from build123d import *

# Parameters (mm, degrees)
ESBO_O1_W                = 18
ESBO_O1_H                = 35
RESSALTO_EXTRUS_O1_DEPTH = 1.5
CORTE_EXTRUS_O1_REACH    = 21.906
ESBO_O2_W                = 13
ESBO_O2_H                = 23
CORTE_EXTRUS_O2_REACH    = 21.906
ESBO_O3_R                = 0.85
FILETE1_R                = 2
ESBO_O4_W                = 3
ESBO_O4_H                = 10
RESSALTO_EXTRUS_O2_DEPTH = 5.73
RESSALTO_EXTRUS_O2_DRAFT = -8
ESBO_O5_W                = 18.610597966
ESBO_O5_H                = 11.610597966
RESSALTO_EXTRUS_O3_DEPTH = 2
CORTE_EXTRUS_O4_REACH    = 46.648
ESBO_O7_R                = 1.75


with BuildPart() as part:
    # Esboço1 → Ressalto-extrusão1 (new, symmetric)
    with BuildSketch(Plane(origin=(0, 0, 0), x_dir=(0, 0, -1), z_dir=(1, 0, 0))):
        Rectangle(ESBO_O1_W, ESBO_O1_H)
    extrude(amount=RESSALTO_EXTRUS_O1_DEPTH, both=True)

    # Esboço2 → Corte-extrusão1 (cut, up to next)
    with BuildSketch(Plane(origin=(1.5, 0, 0), x_dir=(0, 0, -1), z_dir=(1, 0, 0)), mode=Mode.PRIVATE) as corte_extrus_o1_sk1:
        Rectangle(ESBO_O2_W, ESBO_O2_H)
    corte_extrus_o1_tool1 = extrude(corte_extrus_o1_sk1.sketch, amount=-CORTE_EXTRUS_O1_REACH, mode=Mode.PRIVATE) & part.part
    add(corte_extrus_o1_tool1.solids().sort_by_distance((1.5, 0, 0))[0], mode=Mode.SUBTRACT)

    # Esboço3 → Corte-extrusão2 (cut, up to next)
    with BuildSketch(Plane.ZY.offset(1.5), mode=Mode.PRIVATE) as corte_extrus_o2_sk1:
        with Locations((0, 14)):
            Circle(ESBO_O3_R)
    corte_extrus_o2_tool1 = extrude(corte_extrus_o2_sk1.sketch, amount=-CORTE_EXTRUS_O2_REACH, mode=Mode.PRIVATE) & part.part
    # Esboço3 → Corte-extrusão2 (cut, up to next)
    with BuildSketch(Plane.ZY.offset(1.5), mode=Mode.PRIVATE) as corte_extrus_o2_sk2:
        with Locations((0, -14)):
            Circle(ESBO_O3_R)
    corte_extrus_o2_tool2 = extrude(corte_extrus_o2_sk2.sketch, amount=-CORTE_EXTRUS_O2_REACH, mode=Mode.PRIVATE) & part.part
    add(corte_extrus_o2_tool1.solids().sort_by_distance((-1.5, 14, 0))[0], mode=Mode.SUBTRACT)
    add(corte_extrus_o2_tool2.solids().sort_by_distance((-1.5, -14, 0))[0], mode=Mode.SUBTRACT)

    # Filete1
    filete1_edges = [part.edges().sort_by_distance(p)[0] for p in [
        (0, -17.5, -9),
        (0, -17.5, 9),
        (0, 17.5, 9),
        (0, 17.5, -9),
    ]]
    fillet(filete1_edges, radius=FILETE1_R)


with BuildPart() as ressalto_extrus_o2_tool:
    # Esboço4 → Ressalto-extrusão2 (with draft: the straight prism first)
    with BuildSketch(Plane.XZ.offset(17.5)):
        Rectangle(ESBO_O4_W, ESBO_O4_H)
    extrude(amount=RESSALTO_EXTRUS_O2_DEPTH)
    # Ressalto-extrusão2: the draft: its side faces are tilted about the plane it starts from
    ressalto_extrus_o2_sides = [ressalto_extrus_o2_tool.faces().sort_by_distance(p)[0] for p in [
        (0, -20.365, -5),
        (1.5, -20.365, 0),
        (0, -20.365, 5),
        (-1.5, -20.365, 0),
    ]]
    draft(ressalto_extrus_o2_sides, Plane.XZ.offset(17.5), RESSALTO_EXTRUS_O2_DRAFT)


with BuildPart() as part_1:
    add(part.part)

    # Ressalto-extrusão2: add ressalto_extrus_o2_tool
    add(ressalto_extrus_o2_tool.part)

    # Esboço5 → Ressalto-extrusão3 (add)
    with BuildSketch(Plane.XZ.offset(23.23)):
        Rectangle(ESBO_O5_W, ESBO_O5_H)
    extrude(amount=RESSALTO_EXTRUS_O3_DEPTH)

    # Esboço7 → Corte-extrusão4 (cut, up to next)
    with BuildSketch(Plane.XZ.offset(25.23), mode=Mode.PRIVATE) as corte_extrus_o4_sk1:
        with Locations(Location((-5.805298983, 0, 0), (0, 0, 270))):
            Circle(ESBO_O7_R)
    corte_extrus_o4_tool1 = extrude(corte_extrus_o4_sk1.sketch, amount=-CORTE_EXTRUS_O4_REACH, mode=Mode.PRIVATE) & part_1.part
    # Esboço7 → Corte-extrusão4 (cut, up to next)
    with BuildSketch(Plane.XZ.offset(25.23), mode=Mode.PRIVATE) as corte_extrus_o4_sk2:
        with Locations(Location((5.805298983, 0, 0), (0, 0, 270))):
            Circle(ESBO_O7_R)
    corte_extrus_o4_tool2 = extrude(corte_extrus_o4_sk2.sketch, amount=-CORTE_EXTRUS_O4_REACH, mode=Mode.PRIVATE) & part_1.part
    add(corte_extrus_o4_tool1.solids().sort_by_distance((-5.805299, -25.23, 0))[0], mode=Mode.SUBTRACT)
    add(corte_extrus_o4_tool2.solids().sort_by_distance((5.805299, -25.23, 0))[0], mode=Mode.SUBTRACT)


solid = part_1.part
Could you check a few things on this model? Use its own coordinates, in mm. A direction names the side the tool comes from. Round coordinates to 2 decimals unless told otherwise and drop trailing zeros. Loops run counter-clockwise (first coordinate to the right, second up) from the corner with the lowest first, then second, coordinate; pieces in that order, holes last. Notation, with made-up numbers: (72.5, -16.75) - (79.5, -16.75) arc R22 ccw to (79.5, -0.75) - close; hole circle Ø1 at (-29.5, 7.5). An arc over 180 degrees is marked (long way). Write item = value, one per line.
1) If we mould it in two halves opening along Y, with no side actions, what happens to faces 6 (the cylindrical face through (-0.021, 14.843, -0.111)), 7 (the cylindrical face through (0.02, -16.93, -8.4)), 8 (the flat face through (1.5, 4, 8))? For each: pulls with the +Y half, pulls with the -Y half, needs draft (parallel to the pull), parting line crosses it, or undercut.
Computed:
face_6 = undercut
face_7 = pulls with the -Y half
face_8 = needs draft
2) Imagine slicing it at B-B (y = -4.5). Please give me the cut outline in (x, z).
Computed:
outline = (-1.5, -9) - (1.5, -9) - (1.5, -6.5) - (-1.5, -6.5) - close; (-1.5, 6.5) - (1.5, 6.5) - (1.5, 9) - (-1.5, 9) - close
3) Imagine slicing it at D-D (z = 3.5). Please give me the cut outline in (x, y).
Computed:
outline = (-9.31, -25.23) - (9.31, -25.23) - (9.31, -23.23) - (2.31, -23.23) - (1.5, -17.5) - (1.5, -11.5) - (-1.5, -11.5) - (-1.5, -17.5) - (-2.31, -23.23) - (-9.31, -23.23) - close; (-1.5, 11.5) - (1.5, 11.5) - (1.5, 17.5) - (-1.5, 17.5) - close
4) On a 3-axis mill with a long thin cutter (end or side, diameter ignored), from which of +Z, -Z, +X, -X, +Y, -Y can I reach the whole of each face in a straight line? I mean faces 1 (the flat face through (0, 0, -6.5)), 2 (the flat face through (0, -17.5, 6)), 3 (the flat face through (-1.5, 4, 8)), 4 (the flat face through (0, -17.5, -6)), 5 (the flat face through (7.3, -23.23, 1.4)). Say none if no direction works.
Computed:
face_1 = +X, -X
face_2 = +Z, +X, -X
face_3 = +Z, -Z, -X, +Y
face_4 = -Z, +X, -X
face_5 = +Z, -Z, +X, +Y
5) I need wall thicknesses on line 1 along X through (y, z) = (-24.05, 0); line 2 along Y through (x, z) = (0.15, 0); line 3 along Y through (x, z) = (0, -4.25). Which ranges of each line are inside material? Lowest first, please. Write a range as from..to.
Computed:
line_1 = -9.31..-7.56, -4.06..4.06, 7.56..9.31
line_2 = -25.23..-14.85, -13.15..-11.5, 11.5..13.15, 14.85..17.5
line_3 = -25.23..-11.5, 11.5..17.5
6) I'm going to push flat-ended pins straight in: P1, Ø2.5, axis at y = -14, z = 0, coming from the -X side; P2, Ø1.6, axis at x = -1.5, y = -24, coming from the -Z side; P3, Ø2, axis at x = -2, y = -24, coming from the +Z side. Where does each tip first touch, or does it pass through?
Computed:
P1 = -1.5
P2 = -5.81
P3 = 5.81
7) Imagine slicing it at C-C (x = -0.5). Please give me the cut outline in (y, z).
Computed:
outline = (-25.23, -5.81) - (-23.23, -5.81) - (-17.5, -5) - (-17.5, -7) arc R2 ccw to (-15.5, -9) - (15.5, -9) arc R2 ccw to (17.5, -7) - (17.5, 7) arc R2 ccw to (15.5, 9) - (-15.5, 9) arc R2 ccw to (-17.5, 7) - (-17.5, 5) - (-23.23, 5.81) - (-25.23, 5.81) - close; hole circle Ø1.7 at (-14, 0); hole (-11.5, -6.5) - (11.5, -6.5) - (11.5, 6.5) - (-11.5, 6.5) - close; hole circle Ø1.7 at (14, 0)
8) Imagine slicing it at A-A (z = 0). Give the number of separate pieces and of enclosed holes in the cut face, and give its area (3 significant figures).
Computed:
separate_pieces = 6
enclosed_holes = 0
area = 70.8 mm2
